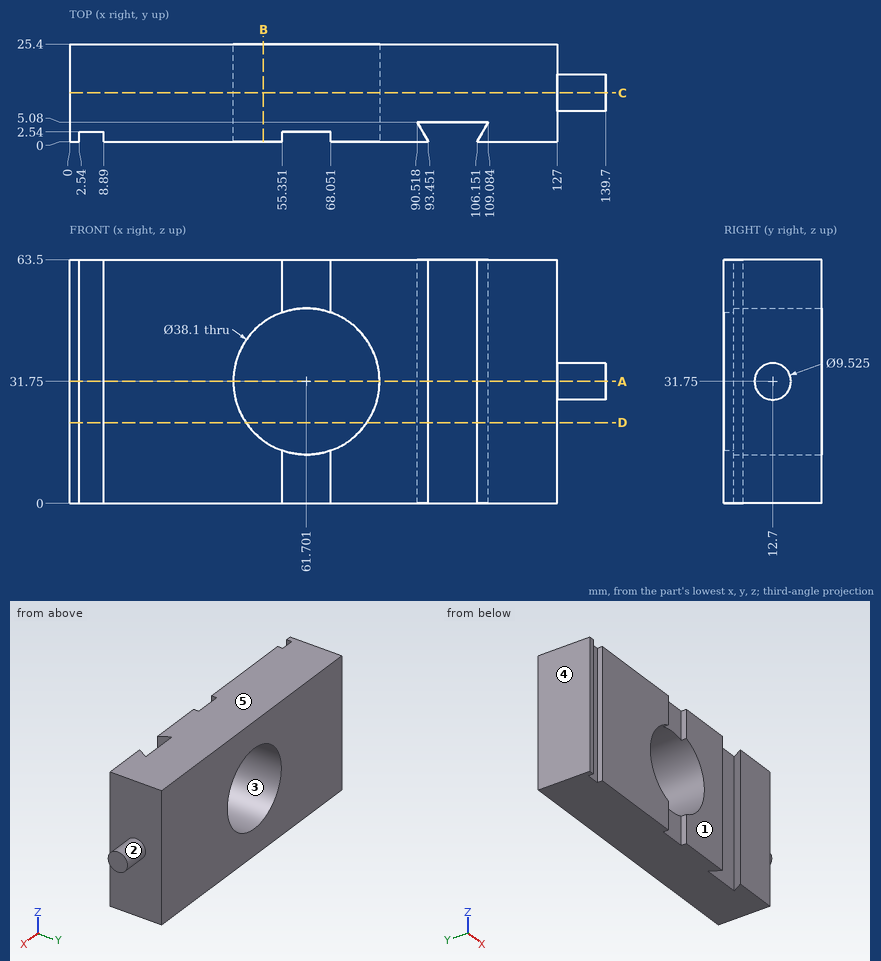
Design review of the part shown in the three views and the two pictorial views. Dimensions are in mm from the part's minimum x, y and z. A direction names the side the tool comes from. Give positions to 0.01 mm unless a question says otherwise; leave off trailing zeros. Loops run counter-clockwise (first coordinate to the right, second up) from the corner with the lowest first, then second, coordinate; pieces in that order, holes last. Notation, with made-up numbers: (35.25, 63.25) -> (39.25, 63.25) arc R31 cw to (39.25, 98.25) -> close; hole circle Ø8 at (72.25, 66). An arc over 180 degrees is marked (long way). Write each question's results on one line, items separated by ' | '.
Q1. Wall thickness on L1, parallel to X at y = 7, z = 31.75; L2, parallel to X at y = 12.5, z = 31.75; L3, parallel to X at y = 16, z = 3.5: over which ranges is each line inside the solid? List them lowest first.
Reply:
L1: x = 0 to 42.65, 80.75 to 127 | L2: x = 0 to 42.65, 80.75 to 139.7 | L3: x = 0 to 127
Q2. The part is to be moulded in two halves that separate along Z. For the marked faces 3, 4 and 5, say which applies: +Z half, -Z half, draft (parallel to the pull), parting line (faces both ways), or undercut.
Reply:
face 3: undercut | face 4: draft | face 5: +Z half
Q3. Take a section at C-C, the plane y = 12.7. Write out the cut boundary in (x, z).
Reply:
outline: (0, 0) -> (127, 0) -> (127, 26.99) -> (139.7, 26.99) -> (139.7, 36.51) -> (127, 36.51) -> (127, 63.5) -> (0, 63.5) -> close; hole circle Ø38.1 at (61.7, 31.75)
Q4. Take a section at D-D, the plane z = 21. Write out the cut boundary in (x, y).
Reply:
outline: (0, 0) -> (2.54, 0) -> (2.54, 2.54) -> (8.89, 2.54) -> (8.89, 0) -> (45.97, 0) -> (45.97, 25.4) -> (0, 25.4) -> close; (77.43, 0) -> (93.45, 0) -> (90.52, 5.08) -> (109.08, 5.08) -> (106.15, 0) -> (127, 0) -> (127, 25.4) -> (77.43, 25.4) -> close
Q5. Take a section at B-B, the plane x = 50.5. Write out the cut boundary in (y, z).
Reply:
outline: (0, 0) -> (25.4, 0) -> (25.4, 16.34) -> (0, 16.34) -> close; (0, 47.16) -> (25.4, 47.16) -> (25.4, 63.5) -> (0, 63.5) -> close
Q6. Machinability: for the marked faces 1 and 2, which of the approach directions +Z, -Z, +X, -X, +Y, -Y give a long, thin tool a straight path to every point of the face, cutting with its end or side? Answer none if there is none.
Reply:
face 1: +Z, -Z, +X, -X, -Y | face 2: +X
Q7. Take a section at A-A, the plane z = 31.75. Write out the cut boundary in (x, y).
Reply:
outline: (0, 0) -> (2.54, 0) -> (2.54, 2.54) -> (8.89, 2.54) -> (8.89, 0) -> (42.65, 0) -> (42.65, 25.4) -> (0, 25.4) -> close; (80.75, 0) -> (93.45, 0) -> (90.52, 5.08) -> (109.08, 5.08) -> (106.15, 0) -> (127, 0) -> (127, 7.94) -> (139.7, 7.94) -> (139.7, 17.46) -> (127, 17.46) -> (127, 25.4) -> (80.75, 25.4) -> close
Q8. For pin 1 Ø1 at (y, z) = (15.5, 45) entering from +X; pin 2 Ø10 at (x, z) = (63, 3.5) entering from -Y, all flat-tipped, find the tip position at first contact; note any pin that passes through.
Reply:
pin 1: stops at x = 127 | pin 2: stops at y = 2.54
